Input: dimensioned drawing with shaded views. Units: mm. Origin: part minimum x, y, z. A direction names the side the tool comes from. Give positions to 0.01 mm unless a question says otherwise; leave off trailing zeros. Order: outer loops, then holes, each group sorted by start corner. A loop starts at its lowest first (then second) coordinate and runs counter-clockwise, first axis right, second up. Notation, with made-up numbers: M 22.5,71.25 L 63.5,71.25 A21 ccw 63.5,87.25 Z; hole C 18.25,58 d1. An arc over 180 degrees is marked long. Answer in a Markdown table with one row per item. Add a question column.
(1) Section query C-C, the plane z = 9. Return loops of the section in (x, y).
(2) Section query A-A, the plane x = 50. Return loops of the section in (y, z).
(3) Section query D-D, the plane z = 28. Return loops of the section in (x, y) (1 decimal), plus the area to 3 significant figures.
(4) Section query B-B, the plane y = 40. Return loops of the section in (x, z), plus the area to 3 significant figures.
(5) Mould query, pull axis Y, two halves, no side actions, for the marked faces 1, 2 and 3. Classes: pulls with the +Y half, pulls with the -Y half, needs draft (parallel to the pull), parting line crosses it, or undercut.
(6) Set-up query: the marked faces 4 and 5. Return all of +Z, -Z, +X, -X, +Y, -Y with unobstructed straight access to the full face (end or side cutting, diameter ignored); none if empty.
(7) Material intervals for line 1 along Y through (x, z) = (50, 22); line 2 along Y through (x, z) = (50, 27); line 3 along X through (y, z) = (40, 16.5), sorted ascending.
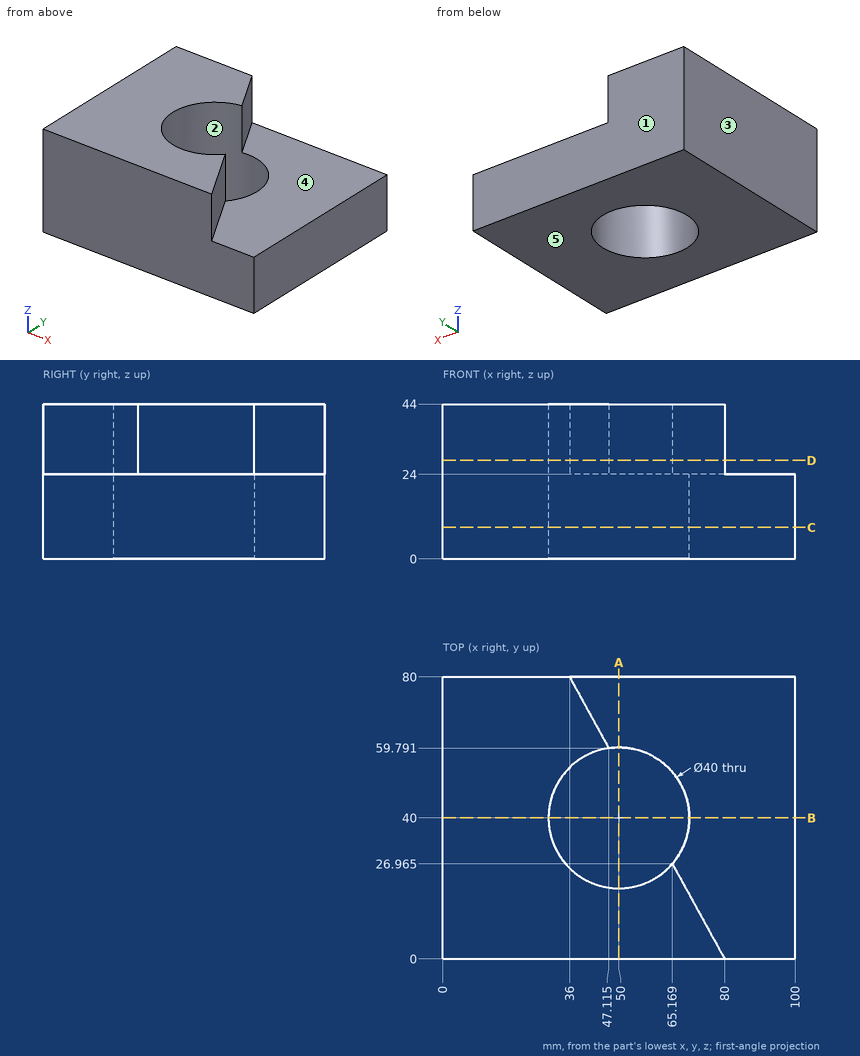
Values follow:
| question | item | result |
|---|---|---|
| 1 | outline | M 0,0 L 100,0 L 100,80 L 0,80 Z; hole C 50,40 d40 |
| 2 | outline | M 0,0 L 20,0 L 20,44 L 0,44 Z; M 60,0 L 80,0 L 80,24 L 60,24 Z |
| 3 | outline | M 0,0 L 80,0 L 65.2,27 A20 cw long 47.1,59.8 L 36,80 L 0,80 Z |
| 3 | area | 3,740 mm² |
| 4 | outline | M 0,0 L 30,0 L 30,44 L 0,44 Z; M 70,0 L 100,0 L 100,24 L 70,24 Z |
| 4 | area | 2,040 mm² |
| 5 | face 1 | pulls with the +Y half |
| 5 | face 2 | undercut |
| 5 | face 3 | needs draft |
| 6 | face 4 | +Z, +X, +Y |
| 6 | face 5 | -Z, +X, -X, +Y, -Y |
| 7 | line 1 | y = 0 to 20, 60 to 80 |
| 7 | line 2 | y = 0 to 20 |
| 7 | line 3 | x = 0 to 30, 70 to 100 |
